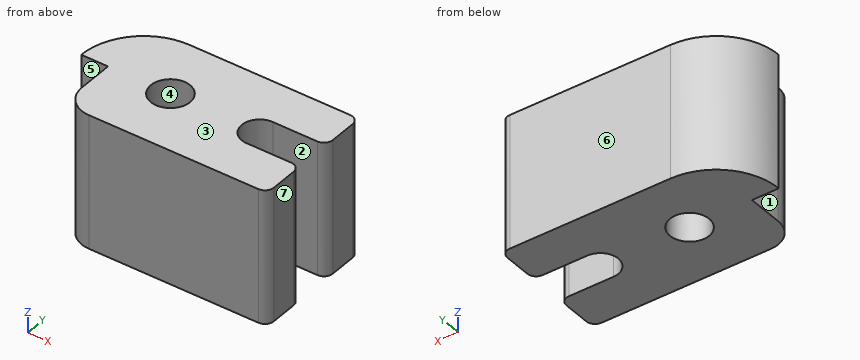
from build123d import *

# Parameters (mm, degrees)
SKETCH1_R           = 2.794
BOSS_EXTRUDE1_DEPTH = 19.05
FILLET2_R           = 8.89
FRONT_FILLET_R      = 1.27
FILLET3_R           = 3.81


with BuildPart() as part:
    # Sketch1 → Boss-Extrude1 (new body)
    with BuildSketch(Plane.XY):
        with BuildLine():
            Line((-12.7, 0), (-8.89, 0))
            Line((-8.89, 0), (-8.89, -8.89))
            Line((-8.89, -8.89), (20.32, -8.89))
            Line((20.32, -8.89), (20.32, -2.54))
            Line((20.32, -2.54), (12.7, -2.54))
            ThreePointArc((12.7, -2.54), (10.16, 0), (12.7, 2.54))
            Line((12.7, 2.54), (20.32, 2.54))
            Line((20.32, 2.54), (20.32, 8.89))
            Line((20.32, 8.89), (-12.7, 8.89))
            Line((-12.7, 8.89), (-12.7, 0))
        make_face()
        with Locations(Location((0, 0, 0), (0, 0, 180))):
            Circle(SKETCH1_R, mode=Mode.SUBTRACT)
    extrude(amount=BOSS_EXTRUDE1_DEPTH)

    # Fillet2
    fillet2_edges = [part.edges().sort_by_distance(p)[0] for p in [
        (-12.7, 8.89, 9.525),
    ]]
    fillet(fillet2_edges, radius=FILLET2_R - 0.0001)  # a hair under: the kernel refuses the full size

    # front_fillet
    front_fillet_edges = [part.edges().sort_by_distance(p)[0] for p in [
        (20.32, -8.89, 9.525),
        (20.32, 8.89, 9.525),
        (20.32, 2.54, 9.525),
        (20.32, -2.54, 9.525),
    ]]
    fillet(front_fillet_edges, radius=FRONT_FILLET_R)

    # Fillet3
    fillet3_edges = [part.edges().sort_by_distance(p)[0] for p in [
        (-8.89, -8.89, 9.525),
    ]]
    fillet(fillet3_edges, radius=FILLET3_R)


solid = part.part
Can you work these out from the model? Positions are in its coordinate system, mm. Face numbers are marked on the shaded views. A direction names the side the tool comes from. Give positions to 0.01 mm unless a question says otherwise; leave off trailing zeros. Loops run counter-clockwise (first coordinate to the right, second up) from the corner with the lowest first, then second, coordinate; pieces in that order, holes last. Notation, with made-up numbers: (58, 10.5) - (107, 10.5) arc R28 ccw to (107, 33.5) - close; hole circle Ø8 at (-20, 71). An arc over 180 degrees is marked (long way). Return JSON: item names as keys, results as strings.
1. I want a section at C-C on y = -1.5. Please give me the cut outline in (x, z).
Output values:
{"outline": "(-8.89, 0) - (-2.36, 0) - (-2.36, 19.05) - (-8.89, 19.05) - close; (2.36, 0) - (10.65, 0) - (10.65, 19.05) - (2.36, 19.05) - close"}
2. I'm going to push flat-ended pins straight in: pin 1 Ø1.5 at (x, z) = (-7, 2.5) entering from +Y; pin 2 Ø1.9 at (x, z) = (-10, 12) entering from -Y; pin 3 Ø4 at (y, z) = (-3, 9.5) entering from -X; pin 4 Ø4.5 at (x, y) = (0, 0) entering from -Z. Where does each tip first touch, or does it pass through?
Output values:
{"pin 1": "stops at y = 8.55", "pin 2": "stops at y = 0", "pin 3": "stops at x = -8.89", "pin 4": "passes through"}
3. I want a section at D-D on y = -6.5. Please give me the cut outline in (x, z).
Output values:
{"outline": "(-8.62, 0) - (20.32, 0) - (20.32, 19.05) - (-8.62, 19.05) - close"}
4. I want a section at B-B on x = 0. Please give me the cut outline in (y, z).
Output values:
{"outline": "(-8.89, 0) - (-2.79, 0) - (-2.79, 19.05) - (-8.89, 19.05) - close; (2.79, 0) - (8.89, 0) - (8.89, 19.05) - (2.79, 19.05) - close"}
5. We'd pull the mould along Y, two halves only. Please class the marked faces 4, 5, 6 and 7: +Y half, -Y half, draft (parallel to the pull), parting line (faces both ways), or undercut.
Output values:
{"face 4": "undercut", "face 5": "-Y half", "face 6": "+Y half", "face 7": "draft"}
6. If I drill on line 1 (Y direction, x = 0, z = 12.75); line 2 (Y direction, x = 13.5, z = 7); line 3 (X direction, y = 0.25, z = 7.5), over which ranges is the centre line in solid material (lowest first)?
Output values:
{"line 1": "y = -8.89 to -2.79, 2.79 to 8.89", "line 2": "y = -8.89 to -2.54, 2.54 to 8.89", "line 3": "x = -12.7 to -2.78, 2.78 to 10.17"}
7. For the marked faces 1, 2 and 3, which set-ups out of +Z, -Z, +X, -X, +Y, -Y let a thin tool reach every point of the face, with its end or its side?
Output values:
{"face 1": "+Z, -Z, -X, -Y", "face 2": "+Z, -Z, +X", "face 3": "+Z, +X, -X, +Y, -Y"}
